Geometry check sheet. Reference: the model listing, model coordinates, mm. Coordinates: 2 decimals unless noted, no trailing zeros. Loops run counter-clockwise (first coordinate to the right, second up) from the corner with the lowest first, then second, coordinate; pieces in that order, holes last. Notation, with made-up numbers: M -22.5,-12 L 22.5,-12 A33 ccw 22.5,17 Z; hole C 20,18 d4. An arc over 180 degrees is marked long. Use CSV: the item, a comma, the result in double quotes.
```python
from build123d import *

# Parameters (mm, degrees)
SKETCH_1_R      = 6.75
SKETCH_1_R_2    = 1.25
EXTRUDE_1_DEPTH = 2


with BuildPart() as part:
    # 草图1 → 凸台-拉伸1 (new body)
    with BuildSketch(Plane(origin=(0, 0, 0), x_dir=(1, 0, 0), z_dir=(0, 1, 0))):
        with BuildLine():
            ThreePointArc((11.093218509, 2.151860383), (-6.318879809, 9.36812457), (-6.150763, -9.479352009))
            ThreePointArc((-6.150763, -9.479352009), (11.261335318, -16.695616197), (11.093218509, 2.151860383))
        make_face()
        Circle(SKETCH_1_R, mode=Mode.SUBTRACT)
        with Locations((-3.132469042, -10.556402687)):
            Circle(SKETCH_1_R_2, mode=Mode.SUBTRACT)
        with Locations((10.961169691, -1.050123328)):
            Circle(SKETCH_1_R_2, mode=Mode.SUBTRACT)
    extrude(amount=EXTRUDE_1_DEPTH)


solid = part.part
```
1. Release check for a two-part mould opening along Z. For faces 1 (the flat face through (2, 0, 7)), 2 (the cylindrical face through (11, 0.986, 16.867)), 3 (the cylindrical face through (-1.46, 0.99, 6.59)) record: +Z half, -Z half, draft (parallel to the pull), parting line (faces both ways), or undercut.
The answers:
face 1,"draft"
face 2,"parting line"
face 3,"undercut"
2. Gauge pin test, flat end, axial feed: P1, Ø1.5, axis at x = 10.96, z = 1.05, coming from the +Y side. Record the tip position at first contact, or that the pin passes through.
The answers:
P1,"through"
3. Thickness scan on line 1 (X direction, y = 0.6, z = 0); line 2 (Z direction, x = -3.5, y = 1.7); line 3 (X direction, y = 0.6, z = 0.25). Record the ranges inside material, lowest first. Write a range as [from, to].
The answers:
line 1,"[-11.3, -6.75], [6.75, 10.28], [11.64, 13.54]"
line 2,"[-10.74, -5.77], [5.77, 9.36], [11.75, 14.84]"
line 3,"[-11.3, -6.75], [6.75, 10], [11.92, 13.75]"
4. Section check C-C, the plane y = 0.6. Record the cut outline in (x, z), plus the area to 3 significant figures.
The answers:
outline,"M -6.15,9.48 A11.3 ccw long 11.09,-2.15 A11.3 ccw long Z; hole C 0,0 d13.5; hole C -3.13,10.56 d2.5; hole C 10.96,1.05 d2.5"
area,"443 mm^2"
5. Section check A-A, the plane x = 0. Record the cut outline in (y, z).
The answers:
outline,"M 0,-11.3 L 2,-11.3 L 2,-6.75 L 0,-6.75 Z; M 0,6.75 L 2,6.75 L 2,17.49 L 0,17.49 Z"
6. Section check B-B, the plane z = 2.75. Record the cut outline in (x, y).
The answers:
outline,"M -10.96,0 L -6.16,0 L -6.16,2 L -10.96,2 Z; M 6.16,0 L 15.27,0 L 15.27,2 L 6.16,2 Z"
7. Section check D-D, the plane x = -9. Record the cut outline in (y, z), plus the area to 3 significant figures.
The answers:
outline,"M 0,-6.83 L 2,-6.83 L 2,6.83 L 0,6.83 Z"
area,"27.3 mm^2"
